Study the drawing (mm; zero at the part's minimum x, y, z) and answer. Give positions to 0.01 mm unless a question says otherwise; leave off trailing zeros. Order: outer loops, then holes, each group sorted by start corner. A loop starts at its lowest first (then second) coordinate and runs counter-clockwise, first axis right, second up. Notation, with made-up numbers: (81.25, 8) - (106.25, 8) arc R27 cw to (106.25, 30) - close; hole circle Ø1 at (20.5, 61.5). An arc over 180 degrees is marked (long way). Write each question's results on one line, items separated by ' | '. Start each with the question number.
1. A flat-ended cylindrical pin translates along its axis: pin 1 (0.6 mm diameter, centred on x = 56.5, z = 1, fed in from +Y). Find the tip coordinate at first contact, or state that the pin passes through.
2. Find the intervals of material crossed by L1, parallel to X at y = 13, z = 1.4; L2, parallel to Y at x = 11, z = 0.55, in increasing order.
3. Section C-C (x = 13) is taken. Give the vertices of the cut face in (y, z).
4. Section A-A (x = 65) is taken. Give the vertices of the cut face in (y, z), and give its area (3 significant figures).
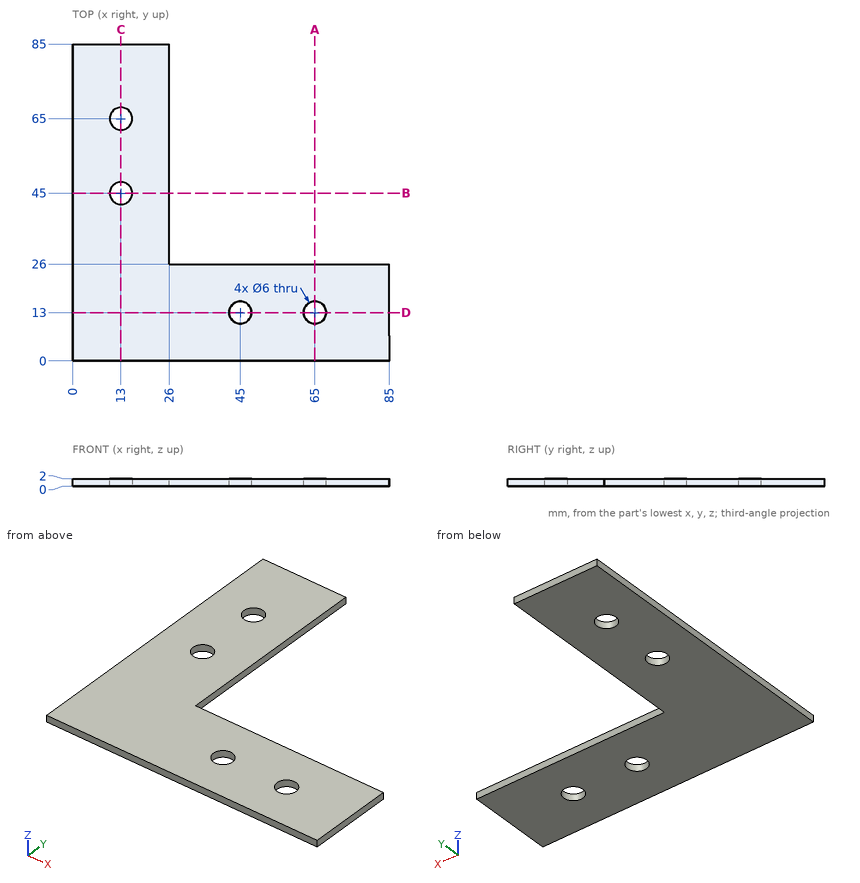
Reported:
1) pin 1: y = 26
2) L1: 0 to 42, 48 to 62, 68 to 85 | L2: 0 to 42.76, 47.24 to 62.76, 67.24 to 85
3) outline: (0, 0) - (42, 0) - (42, 2) - (0, 2) - close; (48, 0) - (62, 0) - (62, 2) - (48, 2) - close; (68, 0) - (85, 0) - (85, 2) - (68, 2) - close
4) outline: (0, 0) - (10, 0) - (10, 2) - (0, 2) - close; (16, 0) - (26, 0) - (26, 2) - (16, 2) - close | area: 40.0 mm²
